from build123d import *

# Parameters (mm, degrees)
F0_R     = 4
F1_DEPTH = 25
F2_DEPTH = 3
F3_DEPTH = 18


with BuildPart() as f1:
    # F0 (on Top) → F1 (new body)
    with BuildSketch(Plane.XY):
        with BuildLine():
            ThreePointArc((-80, -80), (-77.0710678119, -87.0710678119), (-70, -90))
            Line((-70, -90), (70, -90))
            ThreePointArc((70, -90), (77.0710678119, -87.0710678119), (80, -80))
            Line((80, -80), (80, 80))
            ThreePointArc((80, 80), (77.0710678119, 87.0710678119), (70, 90))
            Line((70, 90), (-70, 90))
            ThreePointArc((-70, 90), (-77.0710678119, 87.0710678119), (-80, 80))
            Line((-80, 80), (-80, -80))
        make_face()
        with Locations((-60, -67.5)):
            Circle(F0_R, mode=Mode.SUBTRACT)
        with Locations((60, -67.5)):
            Circle(F0_R, mode=Mode.SUBTRACT)
        with Locations((-60, 67.5)):
            Circle(F0_R, mode=Mode.SUBTRACT)
        with BuildLine():
            ThreePointArc((-64, 40.2934422872), (-62.5820384798, 46.4328484224), (-58.6153846154, 51.3286200352))
            ThreePointArc((-58.6153846154, 51.3286200352), (0, 71.5), (58.6153846154, 51.3286200352))
            ThreePointArc((58.6153846154, 51.3286200352), (62.5820384798, 46.4328484224), (64, 40.2934422872))
            Line((64, 40.2934422872), (64, -40.2934422872))
            ThreePointArc((64, -40.2934422872), (62.5820384798, -46.4328484224), (58.6153846154, -51.3286200352))
            ThreePointArc((58.6153846154, -51.3286200352), (0, -71.5), (-58.6153846154, -51.3286200352))
            ThreePointArc((-58.6153846154, -51.3286200352), (-62.5820384798, -46.4328484224), (-64, -40.2934422872))
            Line((-64, -40.2934422872), (-64, 40.2934422872))
        make_face(mode=Mode.SUBTRACT)
        with Locations((60, 67.5)):
            Circle(F0_R, mode=Mode.SUBTRACT)
        with BuildLine():
            ThreePointArc((58.6153846154, 51.3286200352), (0, 71.5), (-58.6153846154, 51.3286200352))
            ThreePointArc((-58.6153846154, 51.3286200352), (-62.5820384798, 46.4328484224), (-64, 40.2934422872))
            Line((-64, 40.2934422872), (-64, -40.2934422872))
            ThreePointArc((-64, -40.2934422872), (-62.5820384798, -46.4328484224), (-58.6153846154, -51.3286200352))
            ThreePointArc((-58.6153846154, -51.3286200352), (0, -71.5), (58.6153846154, -51.3286200352))
            ThreePointArc((58.6153846154, -51.3286200352), (62.5820384798, -46.4328484224), (64, -40.2934422872))
            Line((64, -40.2934422872), (64, 40.2934422872))
            ThreePointArc((64, 40.2934422872), (62.5820384798, 46.4328484224), (58.6153846154, 51.3286200352))
        make_face()
        with BuildLine():
            Line((-60, -40.2934422872), (-60, 40.2934422872))
            ThreePointArc((-60, 40.2934422872), (-58.9871703427, 44.6787323838), (-56.1538461538, 48.1757121072))
            ThreePointArc((-56.1538461538, 48.1757121072), (0, 67.5), (56.1538461538, 48.1757121072))
            ThreePointArc((56.1538461538, 48.1757121072), (58.9871703427, 44.6787323838), (60, 40.2934422872))
            Line((60, 40.2934422872), (60, -40.2934422872))
            ThreePointArc((60, -40.2934422872), (58.9871703427, -44.6787323838), (56.1538461538, -48.1757121072))
            ThreePointArc((56.1538461538, -48.1757121072), (0, -67.5), (-56.1538461538, -48.1757121072))
            ThreePointArc((-56.1538461538, -48.1757121072), (-58.9871703427, -44.6787323838), (-60, -40.2934422872))
        make_face(mode=Mode.SUBTRACT)
        with BuildLine():
            ThreePointArc((-56.1538461538, 48.1757121072), (-58.9871703427, 44.6787323838), (-60, 40.2934422872))
            Line((-60, 40.2934422872), (-60, -40.2934422872))
            ThreePointArc((-60, -40.2934422872), (-58.9871703427, -44.6787323838), (-56.1538461538, -48.1757121072))
            ThreePointArc((-56.1538461538, -48.1757121072), (0, -67.5), (56.1538461538, -48.1757121072))
            ThreePointArc((56.1538461538, -48.1757121072), (58.9871703427, -44.6787323838), (60, -40.2934422872))
            Line((60, -40.2934422872), (60, 40.2934422872))
            ThreePointArc((60, 40.2934422872), (58.9871703427, 44.6787323838), (56.1538461538, 48.1757121072))
            ThreePointArc((56.1538461538, 48.1757121072), (0, 67.5), (-56.1538461538, 48.1757121072))
        make_face()
        with BuildLine():
            ThreePointArc((54.3076923077, 45.8110311612), (56.2910192399, 43.3631453548), (57, 40.2934422872))
            Line((57, 40.2934422872), (57, -40.2934422872))
            ThreePointArc((57, -40.2934422872), (56.2910192399, -43.3631453548), (54.3076923077, -45.8110311612))
            ThreePointArc((54.3076923077, -45.8110311612), (0, -64.5), (-54.3076923077, -45.8110311612))
            ThreePointArc((-54.3076923077, -45.8110311612), (-56.2910192399, -43.3631453548), (-57, -40.2934422872))
            Line((-57, -40.2934422872), (-57, 40.2934422872))
            ThreePointArc((-57, 40.2934422872), (-56.2910192399, 43.3631453548), (-54.3076923077, 45.8110311612))
            ThreePointArc((-54.3076923077, 45.8110311612), (0, 64.5), (54.3076923077, 45.8110311612))
        make_face(mode=Mode.SUBTRACT)
        with BuildLine():
            Line((57, -40.2934422872), (57, 40.2934422872))
            ThreePointArc((57, 40.2934422872), (56.2910192399, 43.3631453548), (54.3076923077, 45.8110311612))
            ThreePointArc((54.3076923077, 45.8110311612), (0, 64.5), (-54.3076923077, 45.8110311612))
            ThreePointArc((-54.3076923077, 45.8110311612), (-56.2910192399, 43.3631453548), (-57, 40.2934422872))
            Line((-57, 40.2934422872), (-57, -40.2934422872))
            ThreePointArc((-57, -40.2934422872), (-56.2910192399, -43.3631453548), (-54.3076923077, -45.8110311612))
            ThreePointArc((-54.3076923077, -45.8110311612), (0, -64.5), (54.3076923077, -45.8110311612))
            ThreePointArc((54.3076923077, -45.8110311612), (56.2910192399, -43.3631453548), (57, -40.2934422872))
        make_face()
    extrude(amount=-F1_DEPTH)

    # F0 (on Top) → F2 (join)
    with BuildSketch(Plane.XY):
        with BuildLine():
            ThreePointArc((-56.1538461538, 48.1757121072), (-58.9871703427, 44.6787323838), (-60, 40.2934422872))
            Line((-60, 40.2934422872), (-60, -40.2934422872))
            ThreePointArc((-60, -40.2934422872), (-58.9871703427, -44.6787323838), (-56.1538461538, -48.1757121072))
            ThreePointArc((-56.1538461538, -48.1757121072), (0, -67.5), (56.1538461538, -48.1757121072))
            ThreePointArc((56.1538461538, -48.1757121072), (58.9871703427, -44.6787323838), (60, -40.2934422872))
            Line((60, -40.2934422872), (60, 40.2934422872))
            ThreePointArc((60, 40.2934422872), (58.9871703427, 44.6787323838), (56.1538461538, 48.1757121072))
            ThreePointArc((56.1538461538, 48.1757121072), (0, 67.5), (-56.1538461538, 48.1757121072))
        make_face()
        with BuildLine():
            ThreePointArc((54.3076923077, 45.8110311612), (56.2910192399, 43.3631453548), (57, 40.2934422872))
            Line((57, 40.2934422872), (57, -40.2934422872))
            ThreePointArc((57, -40.2934422872), (56.2910192399, -43.3631453548), (54.3076923077, -45.8110311612))
            ThreePointArc((54.3076923077, -45.8110311612), (0, -64.5), (-54.3076923077, -45.8110311612))
            ThreePointArc((-54.3076923077, -45.8110311612), (-56.2910192399, -43.3631453548), (-57, -40.2934422872))
            Line((-57, -40.2934422872), (-57, 40.2934422872))
            ThreePointArc((-57, 40.2934422872), (-56.2910192399, 43.3631453548), (-54.3076923077, 45.8110311612))
            ThreePointArc((-54.3076923077, 45.8110311612), (0, 64.5), (54.3076923077, 45.8110311612))
        make_face(mode=Mode.SUBTRACT)
    extrude(amount=F2_DEPTH)

    # F0 (on Top) → F3 (cut)
    with BuildSketch(Plane.XY):
        with BuildLine():
            Line((57, -40.2934422872), (57, 40.2934422872))
            ThreePointArc((57, 40.2934422872), (56.2910192399, 43.3631453548), (54.3076923077, 45.8110311612))
            ThreePointArc((54.3076923077, 45.8110311612), (0, 64.5), (-54.3076923077, 45.8110311612))
            ThreePointArc((-54.3076923077, 45.8110311612), (-56.2910192399, 43.3631453548), (-57, 40.2934422872))
            Line((-57, 40.2934422872), (-57, -40.2934422872))
            ThreePointArc((-57, -40.2934422872), (-56.2910192399, -43.3631453548), (-54.3076923077, -45.8110311612))
            ThreePointArc((-54.3076923077, -45.8110311612), (0, -64.5), (54.3076923077, -45.8110311612))
            ThreePointArc((54.3076923077, -45.8110311612), (56.2910192399, -43.3631453548), (57, -40.2934422872))
        make_face()
    extrude(amount=-F3_DEPTH, mode=Mode.SUBTRACT)


solid = f1.part
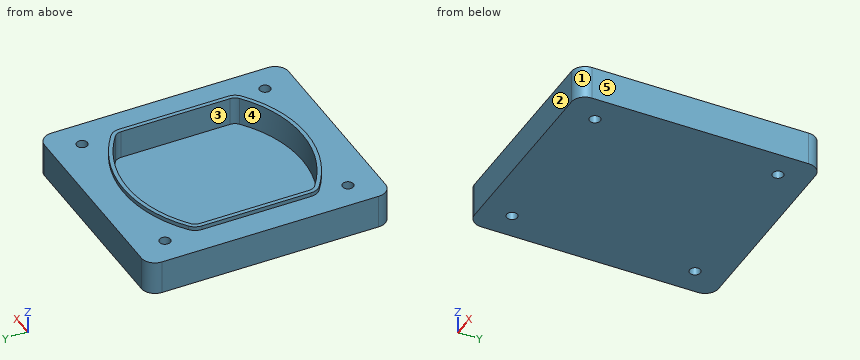
Read the model definition and answer for the solid it produces. Units are mm, in the model's axes. Face numbers are marked on the shaded views. A direction names the side the tool comes from. Coordinates: 2 decimals unless noted, no trailing zeros. Loops run counter-clockwise (first coordinate to the right, second up) from the corner with the lowest first, then second, coordinate; pieces in that order, holes last.
Q1. Which of the six approach directions +Z, -Z, +X, -X, +Y, -Y give full straight-line access (tool end or side, diameter ignored) to the marked faces 4 and 5?
Q2. The part is cut by section B-B on y = 17. Write down the section's boundary in (x, z), and give its area (3 significant figures).
Q3. The mould has two halves that part along X. Classify the marked faces 1, 2 and 3: +X half, -X half, draft (parallel to the pull), parting line (faces both ways), or undercut.
Q4. The part is cut by section C-C on x = 1. Write down the section's boundary in (y, z).
Q5. Each of these flat-tipped pins is pushed along its axis until it touches: pin 1 Ø10.5 at (x, y) = (60, 67.5) entering from -Z; pin 2 Ø10.5 at (x, y) = (60, -67.5) entering from +Z; pin 3 Ø6 at (x, y) = (-15.5, -23) entering from +Z; pin 4 Ø1.5 at (y, z) = (4.5, 1) entering from +X. Where does it stop, or does it pass through?
Q6. Consider probe 1 along Y at (x, z) = (60, -14.75); probe 2 along Y at (x, z) = (-1, -14.5); probe 3 along X at (y, z) = (40.5, 1.5). Determine where each line is inside the solid, lowest interval first.
Q7. The part is cut by section A-A on z = -12. Write down the section's boundary in (x, y), and give its area (3 significant figures).
Results below:
1. face 4: +Z
1. face 5: +Z, -Z, +X, +Y, -Y
2. outline: (-80, -25) - (80, -25) - (80, 0) - (60, 0) - (60, 3) - (57, 3) - (57, -18) - (-57, -18) - (-57, 3) - (-60, 3) - (-60, 0) - (-80, 0) - close
2. area: 1,970 mm2
3. face 1: +X half
3. face 2: draft
3. face 3: undercut
4. outline: (-90, -25) - (90, -25) - (90, 0) - (67.49, 0) - (67.49, 3) - (64.49, 3) - (64.49, -18) - (-64.49, -18) - (-64.49, 3) - (-67.49, 3) - (-67.49, 0) - (-90, 0) - close
5. pin 1: stops at z = -25
5. pin 2: stops at z = 0
5. pin 3: stops at z = -18
5. pin 4: stops at x = 60
6. probe 1: y = -90 to -71.5, -63.5 to 63.5, 71.5 to 90
6. probe 2: y = -90 to -64.49, 64.49 to 90
6. probe 3: x = -60 to -57, 57 to 60
7. outline: (-80, -80) arc R10 ccw to (-70, -90) - (70, -90) arc R10 ccw to (80, -80) - (80, 80) arc R10 ccw to (70, 90) - (-70, 90) arc R10 ccw to (-80, 80) - close; hole circle Ø8 at (-60, -67.5); hole circle Ø8 at (-60, 67.5); hole (-57, -40.29) arc R7 ccw to (-54.31, -45.81) arc R88.25 ccw to (54.31, -45.81) arc R7 ccw to (57, -40.29) - (57, 40.29) arc R7 ccw to (54.31, 45.81) arc R88.25 ccw to (-54.31, 45.81) arc R7 ccw to (-57, 40.29) - close; hole circle Ø8 at (60, -67.5); hole circle Ø8 at (60, 67.5)
7. area: 15,300 mm2
